Read the model definition and answer for the solid it produces. Units are mm, in the model's axes. A direction names the side the tool comes from. Coordinates: 2 decimals unless noted, no trailing zeros. Loops run counter-clockwise (first coordinate to the right, second up) from the corner with the lowest first, then second, coordinate; pieces in that order, holes last. Notation, with made-up numbers: M 79.5,73.25 L 133.5,73.25 A28 cw 133.5,110.25 Z; hole C 89,19 d11. An arc over 180 degrees is marked long. Use one line per item in the form item = value. Start each with the question number.
1. Flat-ended cylindrical pins translate along their axes: pin 1 (1 mm diameter, centred on x = -8, y = 7, fed in from -Z); pin 2 (1.5 mm diameter, centred on x = 2, z = -3.5, fed in from -Y); pin 3 (2.5 mm diameter, centred on x = -0.5, z = -3.5, fed in from +Y). Find the tip coordinate at first contact, or state that the pin passes through.
2. Find the intervals of material crossed by probe 1 along Y at (x, z) = (0, 2.1) (3 decimals); probe 2 along Z at (x, y) = (-3.25, -5); probe 3 along Y at (x, z) = (-2, 1.5), in increasing order. Write a range as [from, to].
3. For a pull along Y with two mould halves and no side action, classify faces 1 (the cylindrical face through (3.515, -1.107, 1.479)), 2 (the flat face through (0, 6, 3)), 3 (the cylindrical face through (-8.797, 20.859, 1.521)) as released by +Y, released by -Y, zero draft, split by the parting line, or undercut.
4. The part is cut by section D-D (y = -4.5). Give the vertices of the cut face in (x, z), plus the area to 3 significant figures.
5. The part is cut by section C-C (z = -1.25). Give the vertices of the cut face in (x, y), plus the area to 3 significant figures.
6. A tool of negligible diameter and unlimited length cuts with its end or side. For faces 4 (the flat face through (0, -9, -2)), 5 (the flat face through (0, -7, -2)), 6 (the flat face through (0, -8, -5)), 7 (the flat face through (-4.5, -8, -2)), 8 (the flat face through (4.5, -8, -2)), from which of +Z, -Z, +X, -X, +Y, -Y can it reach the whole face along a straight path? Write none if from no direction.
7. The part is cut by section B-B (y = 0). Give the vertices of the cut face in (x, z) (3 decimals).
8. The part is cut by section A-A (x = 0). Give the vertices of the cut face in (y, z) (3 decimals), plus the area to 3 significant figures.
Autodesk Inventor part; units mm, degrees
ref_plane "YZ Plane" through (0, 0, 0) normal (1, 0, 0) x (0, 1, 0)
ref_plane "XZ Plane" through (0, 0, 0) normal (0, 1, 0) x (-1, 0, 0)
ref_plane "XY Plane" through (0, 0, 0) normal (0, 0, 1) x (1, 0, 0)
sketch "Sketch1" plane through (0, 0, 0) normal (0, 0, 1) x (1, 0, 0)
  line L0 (-10, -10) -> (10, -10)
  line L1 (10, -10) -> (10, 22)
  line L2 (10, 22) -> (-10, 22)
  line L3 (-10, 22) -> (-10, -10)
  line L4 (6.3, -6.7) -> (-6.3, -6.7) construction
  line L5 (6.3, 6.7) -> (6.3, -6.7) construction
  line L6 (-6.3, 6.7) -> (6.3, 6.7) construction
  line L7 (-6.3, -6.7) -> (-6.3, 6.7) construction
  line L8 (6.45, -6.85) -> (-6.45, -6.85)
  line L9 (-6.45, -6.85) -> (-6.45, 6.85)
  line L10 (-6.45, 6.85) -> (6.45, 6.85)
  line L11 (6.45, 6.85) -> (6.45, -6.85)
  circle A0 centre (0, 0) radius 3.535 construction
  circle A1 centre (0, 0) radius 3.685
  line L12 (4.65, -9.15) -> (-4.65, -9.15) construction
  line L13 (-4.65, -9.15) -> (-4.65, -6.85) construction
  line L14 (-4.65, -6.85) -> (4.65, -6.85) construction
  line L15 (4.65, -6.85) -> (4.65, -9.15) construction
  line L16 (4.5, -7) -> (-4.5, -7)
  line L17 (-4.5, -7) -> (-4.5, -9)
  line L18 (-4.5, -9) -> (4.5, -9)
  line L19 (4.5, -9) -> (4.5, -7)
  point P0 (0, 22)
  point P1 (0, 6.85)
  point P2 (6.45, 0)
  point P3 (0, -6.85)
  point P4 (0, -7)
  point P5 (0, -9)
  point P6 (0, -9.15)
  point P7 (0, -10)
  dimension "d0" = 20
  dimension "d1" = 32
  dimension "d2" = 0.15
  dimension "d3" = 0.15
  dimension "d5" = 7.07
  dimension "d6" = 12.9
  dimension "d7" = 13.7
  dimension "d8" = 22
  dimension "d18" = 2
  dimension "d19" = 2.3
  dimension "d20" = 9
  dimension "d21" = 9.3
  dimension "d22" = 0.85
extrude "Extrusion1" add sketch "Sketch1" along normal blind 3 contours L3 L2 L1 L0 | L19 L18 L17 L16
extrude "Extrusion2" add sketch "Sketch1" along normal blind 3 contours L8 L9 L10 L11
fillet "Fillet1" radius 4 2 edges at (10, 22, 1.5) (-10, 22, 1.5)
extrude "Extrusion3" add sketch "Sketch1" against normal blind 5 contours L19 L18 L17 L16
fillet "Fillet2" radius 0.5 4 edges at (4.5, -7, -2.5) (4.5, -9, -2.5) (-4.5, -7, -2.5) (-4.5, -9, -2.5)
properties part number "Rotary Encoder Mount Mk2"
Computed values:
q1.pin_1 = 0
q1.pin_2 = -9
q1.pin_3 = -7
q2.probe_1 = [-10, -3.685], [3.685, 22]
q2.probe_2 = [0, 3]
q2.probe_3 = [-10, -3.1], [3.1, 22]
q3.face_1 = undercut
q3.face_2 = zero draft
q3.face_3 = released by +Y
q4.outline = M -10,0 L 10,0 L 10,3 L -10,3 Z
q4.area = 60.0 mm²
q5.outline = M -4.5,-8.5 A0.5 ccw -4,-9 L 4,-9 A0.5 ccw 4.5,-8.5 L 4.5,-7.5 A0.5 ccw 4,-7 L -4,-7 A0.5 ccw -4.5,-7.5 Z
q5.area = 17.8 mm²
q6.face_4 = -Z, +X, -X, -Y
q6.face_5 = -Z, +X, -X, +Y
q6.face_6 = -Z, +X, -X, +Y, -Y
q6.face_7 = -Z, -X, +Y, -Y
q6.face_8 = -Z, +X, +Y, -Y
q7.outline = M -10,0 L -3.685,0 L -3.685,3 L -10,3 Z; M 3.685,0 L 10,0 L 10,3 L 3.685,3 Z
q8.outline = M -10,0 L -9,0 L -9,-5 L -7,-5 L -7,0 L -3.685,0 L -3.685,3 L -10,3 Z; M 3.685,0 L 22,0 L 22,3 L 3.685,3 Z
q8.area = 83.9 mm²
